from build123d import *

# Parameters (mm, degrees)
F0_W     = 25.527
F0_H     = 25.527
F0_W_2   = 22.987
F0_H_2   = 22.987
F1_DEPTH = 228.6
F2_R     = 1.905
F3_DEPTH = 25.528
F4_W     = 25.527
F4_H     = 25.527
F4_W_2   = 22.987
F4_H_2   = 22.987
F5_DEPTH = 41.9608


with BuildPart() as f1:
    # F0 (on Top) → F1 (new body)
    with BuildSketch(Plane.XY):
        Rectangle(F0_W, F0_H)
        Rectangle(F0_W_2, F0_H_2, mode=Mode.SUBTRACT)
    extrude(amount=F1_DEPTH)

    # F2 (on face) → F3 (cut, through all)
    with BuildSketch(Plane.XZ.offset(12.7635)):
        with Locations((0, 38.1)):
            Circle(F2_R)
        with Locations((0, 76.2)):
            Circle(F2_R)
        with Locations((0, 114.3)):
            Circle(F2_R)
        with Locations((0, 152.4)):
            Circle(F2_R)
        with Locations((0, 190.5)):
            Circle(F2_R)
    extrude(amount=-F3_DEPTH, mode=Mode.SUBTRACT)

    # F4 (on face) → F5 (join)
    with BuildSketch(Plane(origin=(0, 0, 0), x_dir=(1, 0, 0), z_dir=(0, 0, -1))):
        Rectangle(F4_W, F4_H)
        Rectangle(F4_W_2, F4_H_2, mode=Mode.SUBTRACT)
    extrude(amount=F5_DEPTH)


solid = f1.part
For this review, take the finished solid that the model builds, in its own axes (mm). A direction names the side the tool comes from. Coordinates: 2 decimals unless noted, no trailing zeros. Order: outer loops, then holes, each group sorted by start corner. A loop starts at its lowest first (then second) coordinate and runs counter-clockwise, first axis right, second up. Notation, with made-up numbers: (18, 80.25) - (27, 80.25) arc R9 cw to (27, 88.25) - close; hole circle Ø11 at (64, 34.25). An arc over 180 degrees is marked (long way). Use one line per item in the form item = value.
Q1. For probe 1 along Z at (x, y) = (0, 11.8) (3 decimals); probe 2 along Y at (x, z) = (11, 71), list the stretches that pass through material, from the lowest coordinate up. Write a range as from..to.
Checked values:
probe_1 = -41.961..36.195, 40.005..74.295, 78.105..112.395, 116.205..150.495, 154.305..188.595, 192.405..228.6
probe_2 = -12.76..-11.49, 11.49..12.76
Q2. Consider section C-C (z = 4.5). Give the boundary of the cut face in (x, y).
Checked values:
outline = (-12.76, -12.76) - (12.76, -12.76) - (12.76, 12.76) - (-12.76, 12.76) - close; hole (-11.49, -11.49) - (11.49, -11.49) - (11.49, 11.49) - (-11.49, 11.49) - close
Q3. For faces 5 (the flat face through (0, -11.494, 95)), 6 (the flat face through (-1, -12, 228.6)), list the 3-axis set-ups (+Z, -Z, +X, -X, +Y, -Y) from which the entire face can be reached by the end or side of a thin tool; tool diameter is ignored.
Checked values:
face_5 = +Z, -Z
face_6 = +Z, +X, -X, +Y, -Y
Q4. Consider section A-A (y = -5.75). Give the boundary of the cut face in (x, z), then the cut area to 3 significant figures.
Checked values:
outline = (-12.76, -41.96) - (-11.49, -41.96) - (-11.49, 228.6) - (-12.76, 228.6) - close; (11.49, -41.96) - (12.76, -41.96) - (12.76, 228.6) - (11.49, 228.6) - close
area = 687 mm2
Q5. Draft analysis for pull direction Y (two halves, no side actions). For faces 1 (the flat face through (12.764, 0, 95)), 2 (the flat face through (0, 12.764, 95)), 3 (the flat face through (11.494, 0, 95)), 4 (the flat face through (-11.494, 0, 95)), state which applies: +Y half, -Y half, draft (parallel to the pull), parting line (faces both ways), or undercut.
Checked values:
face_1 = draft
face_2 = +Y half
face_3 = undercut
face_4 = undercut
